Autodesk Inventor part; units mm, degrees
ref_plane "YZ Plane" through (0, 0, 0) normal (1, 0, 0) x (0, 1, 0)
ref_plane "XZ Plane" through (0, 0, 0) normal (0, 1, 0) x (-1, 0, 0)
ref_plane "XY Plane" through (0, 0, 0) normal (0, 0, 1) x (1, 0, 0)
sketch "Sketch1" plane through (0, 0, 0) normal (0, 0, 1) x (1, 0, 0)
  circle A0 centre (-194.945, 6.4301) radius 3.3782
  circle A1 centre (-194.945, 25.4801) radius 3.3782
  circle A2 centre (-144.145, 6.4301) radius 3.3782
  circle A3 centre (-144.145, 25.4801) radius 3.3782
  circle A4 centre (-169.545, 15.9551) radius 14.2875
  line L0 (-254, -1.8249) -> (254, -1.8249) construction
  line L1 (-247.65, 40.5304) -> (247.65, 40.5304) construction
  line L2 (-204.47, -0.5549) -> (-204.47, 32.4651)
  line L3 (-204.47, 32.4651) -> (-134.62, 32.4651)
  line L4 (-134.62, 32.4651) -> (-134.62, -0.5549)
  line L5 (-134.62, -0.5549) -> (-204.47, -0.5549)
  point P0 (0, 0)
extrude "Extrusion1" add sketch "Sketch1" along normal blind 3.175
fillet "Fillet1" radius 6.35 4 edges at (-204.47, 32.4651, 1.5875) (-204.47, -0.5549, 1.5875) (-134.62, 32.4651, 1.5875) (-134.62, -0.5549, 1.5875)
equation "\"d2\" = d1"
properties part number "V5 Shooter Bearing Support Plate" material "Aluminum-6061"
Geometry check sheet. Reference: the model listing, model coordinates, mm. Round coordinates to 2 decimals unless told otherwise and drop trailing zeros. Order: outer loops, then holes, each group sorted by start corner. A loop starts at its lowest first (then second) coordinate and runs counter-clockwise, first axis right, second up. Notation, with made-up numbers: M 46.5,29 L 87.5,29 A24 cw 87.5,40 Z; hole C -24,85 d2. An arc over 180 degrees is marked long. Write each question's results on one line, items separated by ' | '. Start each with the question number.
1. Cross-section at A-A on y = 19. Record the boundary of the cut face in (x, z) (3 decimals), plus the area to 3 significant figures.
2. Draft check along X on faces 1 (the face through (-170, 32.465, 2)), 2 (the face through (-197.435, 4.147, 1.565)), 3 (the face through (-136.431, 30.556, 1.61)). Enter one of: pulls with the +X half, pulls with the -X half, needs draft (parallel to the pull), parting line crosses it, or undercut.
3. Cross-section at C-C on x = -165. Record the boundary of the cut face in (y, z) (3 decimals).
4. Go/stop test with a flat-tipped pin: P1, Ø6, axis at x = -194.94, y = 6.43, coming from the -Z side. Record where the tip stops, or that it passes through.
5. Cross-section at B-B on x = -144. Record the boundary of the cut face in (y, z) (3 decimals), plus the area to 3 significant figures.
6. Cross-section at D-D on z = 1.7. Give the number of separate pieces and of enclosed holes in the cut face, plus the area to 3 significant figures.
7. Material ranges on L1, parallel to Y at x = -159.5, z = 1.7; L2, parallel to Y at x = -169, z = 2.75; L3, parallel to X at y = 22.5, z = 0.9, recorded low to high. Write a range as from..to.
Resolved:
1) outline: M -204.47,0 L -183.504,0 L -183.504,3.175 L -204.47,3.175 Z; M -155.586,0 L -134.62,0 L -134.62,3.175 L -155.586,3.175 Z | area: 133 mm2
2) face 1: needs draft | face 2: undercut | face 3: pulls with the +X half
3) outline: M -0.555,0 L 2.41,0 L 2.41,3.175 L -0.555,3.175 Z; M 29.5,0 L 32.465,0 L 32.465,3.175 L 29.5,3.175 Z
4) P1: through
5) outline: M -0.555,0 L 3.055,0 L 3.055,3.175 L -0.555,3.175 Z; M 9.805,0 L 22.105,0 L 22.105,3.175 L 9.805,3.175 Z; M 28.855,0 L 32.465,0 L 32.465,3.175 L 28.855,3.175 Z | area: 62.0 mm2
6) separate pieces: 1 | enclosed holes: 5 | area: 1,490 mm2
7) L1: -0.55..5.79, 26.12..32.47 | L2: -0.55..1.68, 30.23..32.47 | L3: -204.47..-196.54, -193.35..-182.25, -156.84..-145.74, -142.55..-134.62
